Source: CAD feature listing. Evaluate the final solid. Frame: model axes, mm. Face numbers are marked on the shaded views. Give positions to 0.01 mm unless a question says otherwise; leave off trailing zeros. Loops run counter-clockwise (first coordinate to the right, second up) from the corner with the lowest first, then second, coordinate; pieces in that order, holes last. Notation, with made-up numbers: M -24.5,57 L 13.5,57 A30 ccw 13.5,95 Z; hole C -38.5,67 d2. An arc over 180 degrees is marked long. Answer in a Markdown table with one row per item.
Autodesk Inventor part; units mm, degrees
ref_plane "YZ Plane" through (0, 0, 0) normal (1, 0, 0) x (0, 1, 0)
ref_plane "XZ Plane" through (0, 0, 0) normal (0, 1, 0) x (-1, 0, 0)
ref_plane "XY Plane" through (0, 0, 0) normal (0, 0, 1) x (1, 0, 0)
sketch "Skizze1" plane through (0, 0, 0) normal (0, 0, 1) x (1, 0, 0)
  line L0 (0, 8.7) -> (0, 6)
  line L1 (60, 6) -> (90, 6)
  line L2 (90, 6) -> (90, 0)
  line L3 (90, 0) -> (-0.6001, 0)
  line L4 (-0.4751, 0) -> (2.675, 0)
  line L5 (-0.6001, 0) -> (-0.6001, 8.7)
  line L6 (-0.6001, 8.7) -> (0, 8.7)
  line L7 (60, 6) -> (58.9264, 6)
  line L8 (58.9264, 6) -> (0, 6)
  line L9 (0, -0.1135) -> (0, 1.4755)
  dimension "d0" = 90
  dimension "d1" = 30
  dimension "d2" = 12
  dimension "d9" = 0.6001
  dimension "d10" = 17.4
  dimension "d13" = 1.0736
  dimension "d14" = 12
revolve "Körper" add sketch "Skizze1" angle 360 about axis through (90, 0, 0) along (-1, 0, 0)
sketch "Skizze2" plane through (-0.6001, 0, 0) normal (-1, 0, 0) x (0, 0, 1)
  line L0 (0, 10.9697) -> (9.5, 5.4848)
  line L1 (9.5, 5.4848) -> (9.5, -5.4848)
  line L2 (9.5, -5.4848) -> (0, -10.9697)
  line L3 (0, -10.9697) -> (-9.5, -5.4848)
  line L4 (-9.5, -5.4848) -> (-9.5, 5.4848)
  line L5 (-9.5, 5.4848) -> (0, 10.9697)
  point P0 (0, 0)
  point P1 (0, 0)
  dimension "d11" = 19
extrude "Kopf" add sketch "Skizze2" along normal blind 6.9
sketch "Skizze4" plane through (0, 0, 0) normal (0, 0, 1) x (1, 0, 0)
  line L0 (-7.5001, 9.5) -> (-7.5001, 10.9697)
  line L1 (-7.5001, 10.9697) -> (-6.6516, 10.9697)
  line L2 (-6.6516, 10.9697) -> (-7.5001, 9.5)
  line L3 (-1.1851, 0) -> (0.0049, 0)
  line L4 (-0.6001, 10.9697) -> (-7.5001, 10.9697)
  line L5 (-7.5001, 5.4848) -> (-7.5001, 10.9697)
  dimension "d5" = 30
  dimension "d19" = 19
revolve "Fase1" cut sketch "Skizze4" angle 360 about axis through (-10, 0, 0) along (1, 0, 0)
thread "Gewinde"
chamfer "Fase2" distance 1.0735 distance2 1.0736 1 edges at (90, -6, 0) measured on face at (90, 0.7092, -1.87)
equation "\"d0\" = NLG"
equation "\"d1\" = GEL"
equation "\"d2\" = GD"
equation "\"d10\" = SD2"
equation "\"d14\" = BDM"
equation "\"d11\" = SW"
equation "\"d3\" = KOH - SD"
equation "\"d5\" = ANG1"
equation "\"d19\" = SW0"
equation "\"d15\" = GEL"
equation "\"d6\" = -0.5 * SPD + 0.5 * GD"
equation "\"NLG\" = 90"
equation "\"GD\" = NND"
equation "\"BDM\" = NND"
equation "\"KOH\" = 7.5"
equation "\"GEL\" = 30"
equation "\"SW\" = 19"
equation "\"SW0\" = SW"
equation "\"SPD\" = NND - 1.2269 * TPU"
equation "\"SD2\" = 17.4"
equation "\"SD\" = 0.6"
equation "\"ANG1\" = 30deg"
equation "\"GAL\" = 0.61345 * TPU"
equation "\"GUL\" = 0.61345 * TPU"
equation "\"RR\" = 0.6"
equation "\"TOA\" = 30deg"
equation "\"PTC\" = TPU"
equation "\"GD1\" = THREADDIA - 1.2269 * TPU"
equation "\"TPU\" = 1.75"
equation "\"THREADDIA\" = 12"
equation "\"E0\" = 1.155 * SW"
equation "\"NND\" = 12"
properties part number "DIN 931-1 - M12 x 90"
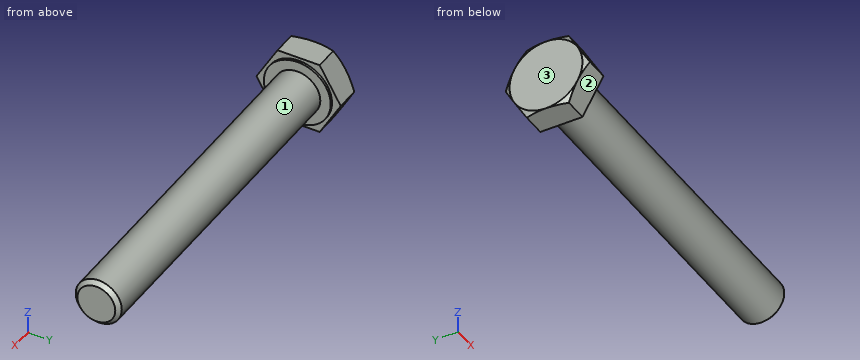
1) Material intervals for L1, parallel to X at y = -8, z = 0.75; L2, parallel to Z at x = 33, y = 0.25; L3, parallel to X at y = 9, z = 1, sorted ascending.
Reply:
| item | result |
|---|---|
| L1 | x = -7.5 to 0 |
| L2 | z = -5.99 to 5.99 |
| L3 | x = -7.5 to -0.6 |
2) Section A-A, the plane x = 67. Return loops of the section in (y, z).
Reply:
| item | result |
|---|---|
| outline | C 0,0 d12 |
3) Pin query (flat end, axial travel): pin 1 Ø10 at (x, z) = (48.5, -1.5) entering from -Y; pin 2 Ø8 at (x, z) = (47, 1) entering from +Y; pin 3 Ø8 at (x, y) = (49.5, -1.5) entering from -Z. Return the tip coordinate at first contact, or that it passes through.
Reply:
| item | result |
|---|---|
| pin 1 | stops at y = -6 |
| pin 2 | stops at y = 6 |
| pin 3 | stops at z = -6 |
4) Pull-direction query (Z, two-part tool) for the marked faces 1, 2 and 3; classes: released by +Z, released by -Z, zero draft, split by the parting line, or undercut.
Reply:
| item | result |
|---|---|
| face 1 | split by the parting line |
| face 2 | released by -Z |
| face 3 | zero draft |
